Here's how the part is built. I have some questions about the finished solid (model axes, mm). Round coordinates to 2 decimals unless told otherwise and drop trailing zeros. Write each loop counter-clockwise with the first axis right and the second up, starting at its lowest first coordinate (ties: lowest second). Pieces come first, ordered by that corner, then holes. Notation, with made-up numbers: (-31, -13.5) - (28, -13.5) arc R32 cw to (28, 25.5) - close; hole circle Ø8 at (14, 1.5). An arc over 180 degrees is marked (long way). Use one line per item in the form item = value. Start each with the question number.
1. I want a section at A-A, the plane y = -1. List the corners of the cut face in (x, z) for me, plus the area to 3 significant figures.
2. We'd pull the mould along X, two halves only. Please class faces 1 (the flat face through (-0.945, -1.375, 3.665)), 2 (the flat face through (0, 0, 0)), 3 (the flat face through (-4, 0, 1)): +X half, -X half, draft (parallel to the pull), parting line (faces both ways), or undercut.
3. If I drill on line 1 along X through (y, z) = (-0.5, 10.25); line 2 along Y through (x, z) = (1.75, 13.5); line 3 along X through (y, z) = (-0.75, 10.75), over which ranges is the centre line in solid material (lowest first)?
4. I want a section at C-C, the plane z = 3. List the corners of the cut face in (x, y) for me, plus the area to 3 significant figures.
5. Will these pins go through, and if not, where does the flat tip stop? pin 1 (2 mm diameter, centred on x = -0.5, z = 6, fed in from +Y); pin 2 (1 mm diameter, centred on x = 0, z = 10, fed in from -Y).
6. I want a section at B-B, the plane x = -2.25. List the corners of the cut face in (y, z) for me, plus the area to 3 significant figures.
```python
from build123d import *

# Parameters (mm, degrees)
F0_W     = 8
F0_H     = 6
F1_DEPTH = 5.08
F3_DEPTH = 25.4
F7_DEPTH = 12.7


with BuildPart() as f1:
    # F0 (on Top) → F1 (new body)
    with BuildSketch(Plane.XY):
        Rectangle(F0_W, F0_H)
    extrude(amount=F1_DEPTH)

    # F2 (on face) → F3 (cut)
    with BuildSketch(Plane.XZ.offset(3)):
        Polygon((-4, 2.7906689793), (4, 5.08), (-4, 5.08), align=None)
    extrude(amount=-F3_DEPTH, mode=Mode.SUBTRACT)

    # F4 (on Front) → F5 (revolve)
    with BuildSketch(Plane.XZ):
        Polygon((2.5232785847, 14.0600437298), (0, 2.9419534787), (1.2592966668, 2.6605941821), (3.8464304525, 14.0600437298), align=None)
    revolve(axis=Axis((1.2616392924, 0, 8.5009986043), (0.221324163, 0, 0.9752002947)))

    # F6 (on Front) → F7 (cut, symmetric)
    with BuildSketch(Plane.XZ):
        Polygon((2.4923852179, 17.2210689634), (-1.6191779869, 13.1095070392), (7.5650927611, 14.7648118436), align=None)
    extrude(amount=F7_DEPTH, both=True, mode=Mode.SUBTRACT)


solid = f1.part
```
Model answer:
q1.outline = (-4, 0) - (4, 0) - (4, 5.08) - (1.14, 4.26) - (3.35, 14) - (1.6, 13.69) - (-0.65, 3.75) - (-4, 2.79) - close
q1.area = 47.9 mm2
q2.face_1 = undercut
q2.face_2 = draft
q2.face_3 = -X half
q3.line_1 = 0.44 to 2.88
q3.line_2 = -1.13 to 1.13
q3.line_3 = 0.7 to 2.85
q4.outline = (-3.27, -3) - (4, -3) - (4, 3) - (-3.27, 3) - close
q4.area = 43.6 mm2
q5.pin_1 = 1.28
q5.pin_2 = -0.73
q6.outline = (-3, 0) - (3, 0) - (3, 3.29) - (-3, 3.29) - close
q6.area = 19.7 mm2
